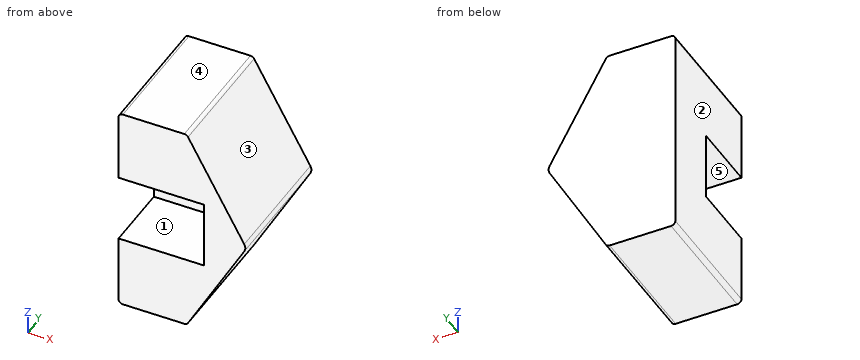
```python
from build123d import *

# Parameters (mm, degrees)
EXTRUDE_1_DEPTH     = 150
SKETCH_2_W          = 80
SKETCH_2_H          = 80
CUT_EXTRUDE_1_DEPTH = 100


with BuildPart() as part:
    # 草图1 → 凸台-拉伸1 (new body)
    with BuildSketch(Plane(origin=(0, 0, 0), x_dir=(1, 0, 0), z_dir=(0, 1, 0))):
        with BuildLine():
            Line((0, -5), (0, -245))
            ThreePointArc((0, -245), (1.464466094, -248.535533906), (5, -250))
            Line((5, -250), (77.069380487, -250))
            ThreePointArc((77.069380487, -250), (79.597711535, -249.313646035), (81.431910567, -247.443016845))
            Line((81.431910567, -247.443016845), (147.351808168, -129.728913986))
            ThreePointArc((147.351808168, -129.728913986), (148.585749894, -125), (147.351808168, -120.271086014))
            Line((147.351808168, -120.271086014), (81.431910567, -2.556983155))
            ThreePointArc((81.431910567, -2.556983155), (79.597711535, -0.686353965), (77.069380487, 0))
            Line((77.069380487, 0), (5, 0))
            ThreePointArc((5, 0), (1.464466094, -1.464466094), (0, -5))
        make_face()
    extrude(amount=EXTRUDE_1_DEPTH)

    # 草图2 → 切除-拉伸1 (cut)
    with BuildSketch(Plane.ZY):
        with Locations((125, 40)):
            Rectangle(SKETCH_2_W, SKETCH_2_H)
    extrude(amount=-CUT_EXTRUDE_1_DEPTH, mode=Mode.SUBTRACT)


solid = part.part
```
The listing builds one solid part. Answer for the finished solid, in the listing's coordinates (mm). Face numbers are marked on the shaded views. A direction names the side the tool comes from. Give positions to 0.01 mm unless a question says otherwise; leave off trailing zeros. Order: outer loops, then holes, each group sorted by start corner. A loop starts at its lowest first (then second) coordinate and runs counter-clockwise, first axis right, second up. Notation, with made-up numbers: M 43,-6 L 96,-6 A34 ccw 96,30 Z; hole C -31.75,21.25 d3. An arc over 180 degrees is marked long. Put each result on its own line as item: value. Start each with the question number.
Item 1: The part is cut by section A-A, the plane y = 69.5. Determine the outline of the cut face in (x, z).
Item 2: The part is cut by section C-C, the plane z = 92.5. Determine the outline of the cut face in (x, y).
Item 3: Find the intervals of material crossed by line 1 along Z through (x, y) = (25.5, 10); line 2 along Y through (x, z) = (59.5, 140.5); line 3 along X through (y, z) = (104.5, 56.5), in increasing order.
Item 4: Which of the six approach directions +Z, -Z, +X, -X, +Y, -Y give full straight-line access (tool end or side, diameter ignored) to the marked faces 4 and 5?
Item 5: The part is cut by section B-B, the plane x = 36. Determine the outline of the cut face in (y, z), and give its area (3 significant figures).
Item 6: For a pull along Z with two mould halves and no side action, classify the marked faces 1, 2 and 3 as +Z half, -Z half, draft (parallel to the pull), parting line (faces both ways), or undercut.
Item 7: Flat-ended cylindrical pins translate along their axes: P1, Ø5, axis at y = 73, z = 152.5, coming from the -X side; P2, Ø10, axis at y = 47, z = 195.5, coming from the +X side; P3, Ø3, axis at y = 77, z = 160, coming from the +X side. Find the tip coordinate at first contact, or state that the pin passes through.
Item 8: The part is cut by section D-D, the plane y = 100.5. Determine the outline of the cut face in (x, z).
Answer key:
1. outline: M 0,5 A5 ccw 5,0 L 77.07,0 A5 ccw 81.43,2.56 L 147.35,120.27 A9.68 ccw 147.35,129.73 L 81.43,247.44 A5 ccw 77.07,250 L 5,250 A5 ccw 0,245 L 0,165 L 100,165 L 100,85 L 0,85 Z
2. outline: M 0,80 L 100,80 L 100,0 L 131.8,0 L 131.8,150 L 0,150 Z
3. line 1: z = 0 to 85, 165 to 250
3. line 2: y = 80 to 150
3. line 3: x = 0 to 111.64
4. face 4: +Z, +X, -X, +Y, -Y
4. face 5: -X, -Y
5. outline: M 0,0 L 150,0 L 150,250 L 0,250 L 0,165 L 80,165 L 80,85 L 0,85 Z
5. area: 31,100 mm²
6. face 1: undercut
6. face 2: draft
6. face 3: +Z half
7. P1: stops at x = 100
7. P2: stops at x = 113.32
7. P3: stops at x = 131.24
8. outline: M 0,5 A5 ccw 5,0 L 77.07,0 A5 ccw 81.43,2.56 L 147.35,120.27 A9.68 ccw 147.35,129.73 L 81.43,247.44 A5 ccw 77.07,250 L 5,250 A5 ccw 0,245 Z
